Model file for the job. Use its own axes, mm. A direction names the side the tool comes from. Coordinates: 2 decimals unless noted, no trailing zeros. Order: outer loops, then holes, each group sorted by start corner. A loop starts at its lowest first (then second) coordinate and runs counter-clockwise, first axis right, second up.
from build123d import *

# Parameters (mm, degrees)
SKETCH_2_R          = 2.05
CUT_EXTRUDE_1_DEPTH = 10
SKETCH_3_R          = 1.55
CUT_EXTRUDE_3_DEPTH = 48.428894147
SKETCH_20_R         = 4
CUT_EXTRUDE_4_DEPTH = 29


with BuildPart() as part:
    # 草图1 → 旋转1 (revolve)
    with BuildSketch(Plane(origin=(0, 0, 0), x_dir=(0, 0, -1), z_dir=(1, 0, 0))):
        Polygon((13, 25), (13, 23), (21.25, 23), (21.25, 0), (28.5, 0), (28.5, 3), (22.5, 3), (22.5, 25), align=None)
    revolve(axis=Axis((0, 0, 0), (0, 1, 0)))

    # 草图2 → 切除-拉伸1 (cut)
    with BuildSketch(Plane(origin=(0, 25, 0), x_dir=(1, 0, 0), z_dir=(0, 1, 0))):
        with Locations(Location((0, 17.5, 0), (0, 0, 270))):
            Circle(SKETCH_2_R)
        with Locations(Location((17.5, 0, 0), (0, 0, 270))):
            Circle(SKETCH_2_R)
        with Locations(Location((0, -17.5, 0), (0, 0, 270))):
            Circle(SKETCH_2_R)
        with Locations(Location((-17.5, 0, 0), (0, 0, 270))):
            Circle(SKETCH_2_R)
    extrude(amount=-CUT_EXTRUDE_1_DEPTH, mode=Mode.SUBTRACT)

    # 草图3 → 切除-拉伸3 (cut, through all)
    with BuildSketch(Plane(origin=(0, 0, 0), x_dir=(1, 0, 0), z_dir=(0, 1, 0))):
        with Locations(Location((0, -26.25, 0), (0, 0, 270))):
            Circle(SKETCH_3_R)
        with Locations(Location((-26.25, 0, 0), (0, 0, 270))):
            Circle(SKETCH_3_R)
        with Locations(Location((0, 26.25, 0), (0, 0, 270))):
            Circle(SKETCH_3_R)
        with Locations(Location((26.25, 0, 0), (0, 0, 270))):
            Circle(SKETCH_3_R)
    extrude(amount=CUT_EXTRUDE_3_DEPTH, mode=Mode.SUBTRACT)

    # 草图20 → 切除-拉伸4 (cut)
    with BuildSketch(Plane(origin=(0, 25, 0), x_dir=(1, 0, 0), z_dir=(0, 1, 0))):
        with Locations(Location((-15.909902577, -15.909902577, 0), (0, 0, 320.099688914))):
            Circle(SKETCH_20_R)
    extrude(amount=-CUT_EXTRUDE_4_DEPTH, mode=Mode.SUBTRACT)


solid = part.part
Q1. Probe line 1 (X direction, y = 0.85, z = 0); line 2 (X direction, y = 8, z = 0). List the from-to ranges inside material, lowest first.
Established:
line 1: x = -28.5 to -27.8, -24.7 to -21.25, 21.25 to 24.7, 27.8 to 28.5
line 2: x = -22.5 to -21.25, 21.25 to 22.5
Q2. Cut at C-C, the plane z = -6.5. List the corners of the cut face in (x, y).
Established:
outline: (-27.75, 0) - (-20.23, 0) - (-20.23, 23) - (-11.26, 23) - (-11.26, 25) - (-21.54, 25) - (-21.54, 3) - (-27.75, 3) - close; (11.26, 23) - (20.23, 23) - (20.23, 0) - (27.75, 0) - (27.75, 3) - (21.54, 3) - (21.54, 25) - (11.26, 25) - close
Q3. Cut at D-D, the plane x = 17.5. List the corners of the cut face in (y, z), plus the area to 3 significant figures.
Established:
outline: (0, -22.49) - (3, -22.49) - (3, -14.14) - (25, -14.14) - (25, -2.05) - (23, -2.05) - (23, -12.05) - (0, -12.05) - close; (0, 12.05) - (23, 12.05) - (23, 2.05) - (25, 2.05) - (25, 14.14) - (3, 14.14) - (3, 22.49) - (0, 22.49) - close
area: 195 mm2
Q4. Which spindle directions (+Z, -Z, +X, -X, +Y, -Y) get a long thin tool onto all of the face, cutting with end or side? Do faces 1 (the face through (9, 23, -10)), 2 (the face through (16.556, 14.154, -15.236)), 3 (the face through (-0.594, 1.479, 27.682)). Say none if no direction does.
Established:
face 1: -Y
face 2: +Y
face 3: +Y, -Y
Q5. Drop flat-ended pins along their axis: P1, Ø4.5, axis at x = 17.5, z = 0, coming from the -Y side; P2, Ø5, axis at x = -15.91, z = 15.91, coming from the +Y side; P3, Ø6, axis at y = 11, z = 3.5, coming from the +X side; P4, Ø10, axis at y = 17.5, z = -0.5, coming from the -X side. Give the stop position or say it passes through.
Established:
P1: stops at y = 23
P2: passes through
P3: stops at x = 22.49
P4: stops at x = -22.5
Q6. Cut at B-B, the plane z = 0. Count the separate pieces of the cut face and the enclosed holes in it, plus the area to 3 significant figures.
Established:
separate pieces: 6
enclosed holes: 0
area: 96.5 mm2
Q7. Cut at A-A, the plane x = -26.25. List the corners of the cut face in (y, z).
Established:
outline: (0, -11.1) - (3, -11.1) - (3, -1.55) - (0, -1.55) - close; (0, 1.55) - (3, 1.55) - (3, 11.1) - (0, 11.1) - close
Q8. Mould opens along X. For faces 4 (the face through (0.09, 24.01, 15.45)), 5 (the face through (10.916, 1.521, -26.327)), 6 (the face through (-13, 0, -17)), 7 (the face through (-18.257, 11.632, 12.671)) say: pulls with the +X half, pulls with the -X half, needs draft (parallel to the pull), parting line crosses it, or undercut.
Established:
face 4: undercut
face 5: parting line crosses it
face 6: needs draft
face 7: undercut
